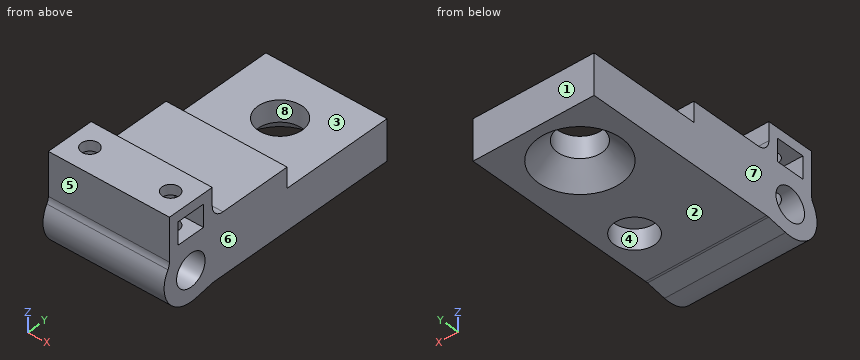
```python
from build123d import *

# Parameters (mm, degrees)
SKETCH1_R                                           = 4
BOSS_EXTRUDE1_DEPTH                                 = 15
SKETCH2_W                                           = 11.5
SKETCH2_H                                           = 12
BOSS_EXTRUDE2_DEPTH                                 = 30
FILLET1_R                                           = 3
SKETCH3_R                                           = 2.1
CUT_EXTRUDE1_DEPTH                                  = 60.211485372
CUT_EXTRUDE2_REACH                                  = 63.662
CUT_EXTRUDE2_END_RADIUS                             = 4
SKETCH4_R                                           = 2.1
CUT_EXTRUDE3_START                                  = -2.5
CUT_EXTRUDE3_DEPTH                                  = 5.5
CUT_EXTRUDE4_DEPTH                                  = 62.288253385
CUT_EXTRUDE4_DEPTH_BACK                             = 5
SKETCH6_R                                           = 5
CSK_FOR_M10_HEX_SOCKET_COUNTERSUNK_HEAD_D           = 11
CSK_FOR_M10_HEX_SOCKET_COUNTERSUNK_HEAD_CSINK_D     = 20.5
CSK_FOR_M10_HEX_SOCKET_COUNTERSUNK_HEAD_CSINK_ANGLE = 90
SKETCH9_W                                           = 30
SKETCH9_H                                           = 28
CUT_EXTRUDE5_DEPTH                                  = 5


with BuildPart() as part:
    # Sketch1 → Boss-Extrude1 (new, symmetric)
    with BuildSketch(Plane(origin=(0, 0, 0), x_dir=(0, 0, -1), z_dir=(1, 0, 0))):
        with BuildLine():
            Line((6.5, 55), (6.5, 6.327446796))
            Line((6.5, 6.327446796), (7.386058148, 1.302361333))
            ThreePointArc((7.386058148, 1.302361333), (1.302361333, -7.386058148), (-7.386058148, -1.302361333))
            Line((-7.386058148, -1.302361333), (-8.5, 5.015116843))
            Line((-8.5, 5.015116843), (-8.5, 55))
            Line((-8.5, 55), (6.5, 55))
        make_face()
        Circle(SKETCH1_R, mode=Mode.SUBTRACT)
    extrude(amount=BOSS_EXTRUDE1_DEPTH, both=True)

    # Sketch2 → Boss-Extrude2 (add)
    with BuildSketch(Plane(origin=(15, 0, 0), x_dir=(0, 0, -1), z_dir=(1, 0, 0))):
        with Locations((-10.25, 0)):
            Rectangle(SKETCH2_W, SKETCH2_H)
    extrude(amount=-BOSS_EXTRUDE2_DEPTH)

    # Fillet1
    fillet1_edges = [part.edges().sort_by_distance(p)[0] for p in [
        (0, 6.327446796, -6.5),
        (0, 6, 8.5),
        (0, -6, 4.5),
    ]]
    fillet(fillet1_edges, radius=FILLET1_R)

    # Sketch3 → Cut-Extrude1 (cut, through all)
    with BuildSketch(Plane.XY.offset(8.5)):
        with Locations((0, 42)):
            Circle(SKETCH3_R)
    extrude(amount=-CUT_EXTRUDE1_DEPTH, mode=Mode.SUBTRACT)

    # Cut-Extrude2: up to this cylinder (the profile starts outside it)
    cut_extrude2_end = Plane(origin=(0, 0, 0), z_dir=(-1, 0, 0)) * Cylinder(CUT_EXTRUDE2_END_RADIUS, 156.324, mode=Mode.PRIVATE)
    # Sketch4 → Cut-Extrude2 (cut, up to the surface)
    with BuildSketch(Plane.XY.offset(16), mode=Mode.PRIVATE) as cut_extrude2_sk1:
        with Locations((-10, 0)):
            Circle(SKETCH4_R)
    cut_extrude2_tool1 = extrude(cut_extrude2_sk1.sketch, amount=-CUT_EXTRUDE2_REACH, mode=Mode.PRIVATE) - cut_extrude2_end
    add(cut_extrude2_tool1.solids().sort_by_distance((-10, 0, 16))[0], mode=Mode.SUBTRACT)
    # Sketch4 → Cut-Extrude2 (cut, up to the surface)
    with BuildSketch(Plane.XY.offset(16), mode=Mode.PRIVATE) as cut_extrude2_sk2:
        with Locations((10, 0)):
            Circle(SKETCH4_R)
    cut_extrude2_tool2 = extrude(cut_extrude2_sk2.sketch, amount=-CUT_EXTRUDE2_REACH, mode=Mode.PRIVATE) - cut_extrude2_end
    add(cut_extrude2_tool2.solids().sort_by_distance((10, 0, 16))[0], mode=Mode.SUBTRACT)

    # Sketch5 → Cut-Extrude3 (cut)
    with BuildSketch(Plane.XY.offset(16).offset(CUT_EXTRUDE3_START)):
        Polygon((-12.049593456, 3.55), (-15, 3.55), (-15, -3.55), (-12.049593456, -3.55), (-7.950406544, -3.55), (-5.900813089, 0), (-7.950406544, 3.55), align=None)
    cut_extrude3 = extrude(amount=-CUT_EXTRUDE3_DEPTH, mode=Mode.SUBTRACT)

    # Mirror1: Cut-Extrude3 across plane
    add(cut_extrude3.mirror(Plane(origin=(0, 0, 0), x_dir=(0, 0, 1), z_dir=(1, 0, 0))), mode=Mode.SUBTRACT)

    # Sketch6 → Cut-Extrude4 (cut, two sides: drawn at the far end of the back side and taken through both)
    with BuildSketch(Plane(origin=(0, 0, -6.5), x_dir=(-1, 0, 0), z_dir=(0, 0, -1)).offset(-CUT_EXTRUDE4_DEPTH_BACK)):
        with Locations(Location((-7, 18.75, 0), (0, 0, 90))):
            Circle(SKETCH6_R)
    extrude(amount=CUT_EXTRUDE4_DEPTH + CUT_EXTRUDE4_DEPTH_BACK, mode=Mode.SUBTRACT)

    # CSK for M10 Hex Socket Countersunk Head Screw1 (through all)
    with Locations(Plane(origin=(0, 0, -6.5), x_dir=(-1, 0, 0), z_dir=(0, 0, -1))):
        with Locations((0, 42)):
            CounterSinkHole(CSK_FOR_M10_HEX_SOCKET_COUNTERSUNK_HEAD_D / 2, CSK_FOR_M10_HEX_SOCKET_COUNTERSUNK_HEAD_CSINK_D / 2, counter_sink_angle=CSK_FOR_M10_HEX_SOCKET_COUNTERSUNK_HEAD_CSINK_ANGLE)

    # Sketch9 → Cut-Extrude5 (cut)
    with BuildSketch(Plane.XY.offset(8.5)):
        with Locations((0, 41)):
            Rectangle(SKETCH9_W, SKETCH9_H)
    extrude(amount=-CUT_EXTRUDE5_DEPTH, mode=Mode.SUBTRACT)


solid = part.part
```
Geometry check sheet. Reference: the model listing, model coordinates, mm. Face numbers are marked on the shaded views. A direction names the side the tool comes from. Coordinates: 2 decimals unless noted, no trailing zeros. Loops run counter-clockwise (first coordinate to the right, second up) from the corner with the lowest first, then second, coordinate; pieces in that order, holes last. Notation, with made-up numbers: (-6.5, -28.75) -> (3.5, -28.75) arc R11 ccw to (3.5, -13.75) -> close; hole circle Ø7 at (38, 40). An arc over 180 degrees is marked (long way). Put each result on its own line as item: value.
1) Release check for a two-part mould opening along X. For the marked faces 6, 7 and 8 record: released by +X, released by -X, zero draft, split by the parting line, or undercut.
Result set:
face 6: released by +X
face 7: released by -X
face 8: undercut
2) Cross-section at A-A on z = 0. Record the boundary of the cut face in (x, y), plus the area to 3 significant figures.
Result set:
outline: (-15, -7.5) -> (15, -7.5) -> (15, -4) -> (-15, -4) -> close; (-15, 4) -> (15, 4) -> (15, 55) -> (-15, 55) -> close; hole circle Ø11 at (0, 42)
area: 1,540 mm^2
3) Cross-section at C-C on x = 13. Record the boundary of the cut face in (y, z).
Result set:
outline: (-6.43, 3.86) arc R7.5 ccw to (1.3, -7.39) -> (6.07, -6.55) arc R3 cw to (6.59, -6.5) -> (55, -6.5) -> (55, 3.5) -> (27, 3.5) -> (27, 8.5) -> (9, 8.5) arc R3 cw to (6, 11.5) -> (6, 16) -> (-6, 16) -> (-6, 5.41) arc R3 cw to start; hole circle Ø8 at (0, 0); hole (-3.55, 8) -> (3.55, 8) -> (3.55, 13.5) -> (-3.55, 13.5) -> close
4) Cross-section at B-B on x = 0. Record the boundary of the cut face in (y, z).
Result set:
outline: (-6.43, 3.86) arc R7.5 ccw to (1.3, -7.39) -> (6.07, -6.55) arc R3 cw to (6.59, -6.5) -> (31.75, -6.5) -> (36.5, -1.75) -> (36.5, 3.5) -> (27, 3.5) -> (27, 8.5) -> (9, 8.5) arc R3 cw to (6, 11.5) -> (6, 16) -> (-6, 16) -> (-6, 5.41) arc R3 cw to start; (47.5, -1.75) -> (52.25, -6.5) -> (55, -6.5) -> (55, 3.5) -> (47.5, 3.5) -> close; hole circle Ø8 at (0, 0)
5) Gauge pin test, flat ends, axial feed: pin 1 Ø1 at (x, z) = (-7, 6.5) entering from -Y; pin 2 Ø9 at (x, y) = (1.5, 35.5) entering from -Z; pin 3 Ø5.5 at (x, y) = (6, 22.5) entering from +Z. Record the tip position at first contact, or that the pin passes through.
Result set:
pin 1: stops at y = -6
pin 2: stops at z = -6.5
pin 3: stops at z = 8.5
6) Tool access check on the marked faces 1, 2, 3, 4 and 5. Record the directions out of +Z, -Z, +X, -X, +Y, -Y that give a thin tool (end or side, any length) a straight path to the whole face; none if there is none.
Result set:
face 1: +Z, -Z, +X, -X, +Y
face 2: -Z, +X, -X, +Y
face 3: +Z, +X, -X, +Y
face 4: -Z
face 5: +Z, +X, -X, -Y
7) Cross-section at D-D on y = -1. Count the separate pieces of the cut face and the enclosed holes in it, plus the area to 3 significant figures.
Result set:
separate pieces: 6
enclosed holes: 0
area: 328 mm^2
8) Thickness scan on line 1 (Z direction, x = -6.5, y = 0); line 2 (X direction, y = 0, z = 5.85); line 3 (X direction, y = 18.75, z = -5.1). Record the ranges inside material, lowest first.
Result set:
line 1: z = -7.5 to -4, 4 to 8, 13.5 to 16
line 2: x = -15 to -12.1, -7.9 to 7.9, 12.1 to 15
line 3: x = -15 to 2, 12 to 15
